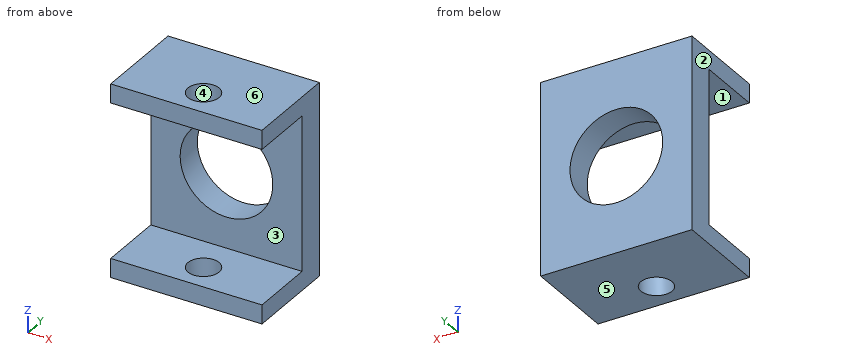
Autodesk Inventor part; units mm, degrees
ref_plane "YZ Plane" through (0, 0, 0) normal (1, 0, 0) x (0, 1, 0)
ref_plane "XZ Plane" through (0, 0, 0) normal (0, 1, 0) x (-1, 0, 0)
ref_plane "XY Plane" through (0, 0, 0) normal (0, 0, 1) x (1, 0, 0)
sketch "Sketch1" plane through (0, 0, 0) normal (0, 1, 0) x (-1, 0, 0)
  circle A0 centre (0, 0) radius 4.9
  circle A1 centre (0, 0) radius 6.9
  line L0 (6.9, 8) -> (-5.9499, 8) construction
  line L1 (6.9, -8) -> (-5.9499, -8) construction
  line L2 (8, 8.15) -> (-8, 8.15)
  line L3 (-8, 8.15) -> (-8, -8.15)
  line L4 (-8, -8.15) -> (8, -8.15)
  line L5 (8, -8.15) -> (8, 8.15)
  line L6 (8, 8.15) -> (8, 10.15)
  line L7 (8, 10.15) -> (-8, 10.15)
  line L8 (-8, 10.15) -> (-8, 8.15)
  line L9 (-8, -8.15) -> (-8, -10.15)
  line L10 (-8, -10.15) -> (8, -10.15)
  line L11 (8, -10.15) -> (8, -8.15)
  point P0 (0, -8.15)
  dimension "d0" = 9.8
  dimension "d1" = 2
  dimension "d2" = 16
  dimension "d3" = 8
  dimension "d4" = 0.15
  dimension "d5" = 0.15
  dimension "d6" = 16
  dimension "d7" = 2
  dimension "d8" = 2
extrude "Extrusion1" add sketch "Sketch1" along normal blind 3 contours A1 | L5 L4 L3 L2 | L2 L8 L7 L6 | L11 L10 L9 L4
extrude "Extrusion2" add sketch "Sketch1" against normal blind 7 contours L2 L8 L7 L6 | L11 L10 L9 L4
sketch "Sketch2" plane through (-8, 3, 10.15) normal (0, 0, 1) x (1, 0, 0)
  circle A0 centre (8, -7) radius 1.65
  line L0 (16, -10) -> (0, -10)
  point P0 (8, -3)
  point P1 (8, -10)
  dimension "d13" = 3.3
  dimension "d14" = 3
extrude "Extrusion3" cut sketch "Sketch2" against normal through all
properties part number "ShaftSyncAdapter" material "ABS Plastic"
Here's how the part is built. I have some questions about the finished solid (model axes, mm). Face numbers are marked on the shaded views. A direction names the side the tool comes from. Coordinates: 2 decimals unless noted, no trailing zeros. Write each loop counter-clockwise with the first axis right and the second up, starting at its lowest first coordinate (ties: lowest second). Pieces come first, ordered by that corner, then holes.
Item 1: I want a section at A-A on x = 0. Write out the boundary of the cut face in (y, z), and give its area (3 significant figures).
Item 2: On a 3-axis mill with a long thin cutter (end or side, diameter ignored), from which of +Z, -Z, +X, -X, +Y, -Y can I reach the whole of each face in a straight line? I mean the marked faces 1 and 2. Say none if no direction works.
Item 3: I want a section at B-B on z = 0. Write out the boundary of the cut face in (x, y).
Item 4: I want a section at C-C on y = -4. Write out the boundary of the cut face in (x, z).
Item 5: I want a section at D-D on x = -6. Write out the boundary of the cut face in (y, z), and give its area (3 significant figures).
Item 6: If we mould it in two halves opening along Z, with no side actions, what happens to the marked faces 3, 4, 5 and 6? For each: +Z half, -Z half, draft (parallel to the pull), parting line (faces both ways), or undercut.
Item 7: If I drill on line 1 (Z direction, x = 0, y = 1.5); line 2 (Z direction, x = -6.75, y = -1); line 3 (Y direction, x = 0, z = -9.4), over which ranges is the centre line in solid material (lowest first)?
Findings below:
1. outline: (-7, -10.15) - (-5.65, -10.15) - (-5.65, -8.15) - (-7, -8.15) - close; (-7, 8.15) - (-5.65, 8.15) - (-5.65, 10.15) - (-7, 10.15) - close; (-2.35, -10.15) - (3, -10.15) - (3, -4.9) - (0, -4.9) - (0, -8.15) - (-2.35, -8.15) - close; (-2.35, 8.15) - (0, 8.15) - (0, 4.9) - (3, 4.9) - (3, 10.15) - (-2.35, 10.15) - close
1. area: 46.3 mm2
2. face 1: +X, -X, -Y
2. face 2: +Z, -Z, -X, +Y, -Y
3. outline: (-8, 0) - (-4.9, 0) - (-4.9, 3) - (-8, 3) - close; (4.9, 0) - (8, 0) - (8, 3) - (4.9, 3) - close
4. outline: (-8, -10.15) - (-1.65, -10.15) - (-1.65, -8.15) - (-8, -8.15) - close; (-8, 8.15) - (-1.65, 8.15) - (-1.65, 10.15) - (-8, 10.15) - close; (1.65, -10.15) - (8, -10.15) - (8, -8.15) - (1.65, -8.15) - close; (1.65, 8.15) - (8, 8.15) - (8, 10.15) - (1.65, 10.15) - close
5. outline: (-7, -10.15) - (3, -10.15) - (3, 10.15) - (-7, 10.15) - (-7, 8.15) - (0, 8.15) - (0, -8.15) - (-7, -8.15) - close
5. area: 88.9 mm2
6. face 3: undercut
6. face 4: draft
6. face 5: -Z half
6. face 6: +Z half
7. line 1: z = -10.15 to -4.9, 4.9 to 10.15
7. line 2: z = -10.15 to -8.15, 8.15 to 10.15
7. line 3: y = -7 to -5.65, -2.35 to 3
